Geometry check sheet. Reference: the model listing, model coordinates, mm. A direction names the side the tool comes from. Round coordinates to 2 decimals unless told otherwise and drop trailing zeros. Order: outer loops, then holes, each group sorted by start corner. A loop starts at its lowest first (then second) coordinate and runs counter-clockwise, first axis right, second up. Notation, with made-up numbers: (3, 82) -> (23, 82) arc R36 ccw to (23, 121) -> close; hole circle Ø2 at (5.25, 13). An arc over 180 degrees is marked (long way). Answer as a JSON object with one key per item and string values. Group by question number.
from build123d import *

# Parameters (mm, degrees)
EXTRUDE_1_DEPTH     = 47.7
CUT_EXTRUDE_1_DEPTH = 10
SKETCH_4_R          = 1.5
CUT_EXTRUDE_2_DEPTH = 10
SKETCH_6_R          = 2.5
CUT_EXTRUDE_4_DEPTH = 3


with BuildPart() as part:
    # 草图1 → 凸台-拉伸1 (new body)
    with BuildSketch(Plane(origin=(0, 0, 0), x_dir=(1, 0, 0), z_dir=(0, 1, 0))):
        Polygon((70.07, 0), (76.07, -6), (94.07, -6), (94.07, 0.5), (84.77, 0.5), (79.27, 6), (0, 6), (-79.27, 6), (-84.77, 0.5), (-94.07, 0.5), (-94.07, -6), (-76.07, -6), (-70.07, 0), align=None)
    extrude(amount=EXTRUDE_1_DEPTH)

    # 草图2 → 切除-拉伸1 (cut)
    with BuildSketch(Plane(origin=(0, 0, -6), x_dir=(-1, 0, 0), z_dir=(0, 0, -1))):
        Polygon((-69.27, 39.7), (-69.27, 8), (-54.27, 8), align=None)
        Polygon((-27.632185319, 39.7), (-62.632185319, 39.7), (-47.632185319, 8), align=None)
        Polygon((-40.537826527, 8), (-6.557580565, 8), (-20.537826527, 39.7), align=None)
        Polygon((-13.980245962, 39.7), (0, 8), (13.980245962, 39.7), align=None)
        Polygon((6.557580565, 8), (40.537826527, 8), (20.537826527, 39.7), align=None)
        Polygon((27.632185319, 39.7), (47.632185319, 8), (62.632185319, 39.7), align=None)
        Polygon((69.27, 39.7), (54.27, 8), (69.27, 8), align=None)
    extrude(amount=-CUT_EXTRUDE_1_DEPTH, mode=Mode.SUBTRACT)

    # 草图4 → 切除-拉伸2 (cut)
    with BuildSketch(Plane(origin=(0, 0, -0.5), x_dir=(-1, 0, 0), z_dir=(0, 0, -1))):
        with Locations((-89.57, 34.7)):
            Circle(SKETCH_4_R)
        with Locations((-89.57, 12.2)):
            Circle(SKETCH_4_R)
        with Locations((89.57, 34.7)):
            Circle(SKETCH_4_R)
        with Locations((89.57, 12.2)):
            Circle(SKETCH_4_R)
    extrude(amount=-CUT_EXTRUDE_2_DEPTH, mode=Mode.SUBTRACT)

    # 草图6 → 切除-拉伸4 (cut)
    with BuildSketch(Plane(origin=(0, 0, -0.5), x_dir=(-1, 0, 0), z_dir=(0, 0, -1))):
        with Locations((-89.57, 34.7)):
            Circle(SKETCH_6_R)
        with Locations((-89.57, 12.2)):
            Circle(SKETCH_6_R)
        with Locations((89.57, 34.7)):
            Circle(SKETCH_6_R)
        with Locations((89.57, 12.2)):
            Circle(SKETCH_6_R)
    extrude(amount=-CUT_EXTRUDE_4_DEPTH, mode=Mode.SUBTRACT)


solid = part.part
Item 1: Set-up check for faces 1 (the cylindrical face through (-87.73, 36.39, 0.98)), 2 (the flat face through (-73.11, 23.52, 3.04)), 3 (the flat face through (-30.678, 23.628, -3.042)): record each of +Z, -Z, +X, -X, +Y, -Y from which the full face is reachable in a straight line by a thin tool's end or side.
Item 2: Sectioned sample at A-A, the plane x = 24.5. Enter the section's corners in (y, z), then the cut area to 3 significant figures.
Item 3: Sectioned sample at B-B, the plane y = 29. Count the separate pieces of the cut face and the enclosed holes in it, then the cut area to 3 significant figures.
Item 4: Thickness scan on L1, parallel to Y at x = -89.57, z = 5.15; L2, parallel to Y at x = -89.57, z = 0.65; L3, parallel to X at y = 4.5, z = 4. Record the ranges inside material, lowest first.
Item 5: Depth check by flat-ended pin: pin 1 Ø6.5 at (x, y) = (89.57, 12.2) entering from -Z; pin 2 Ø5 at (x, y) = (89.57, 12.2) entering from +Z; pin 3 Ø6 at (x, y) = (-16, 26.5) entering from +Z; pin 4 Ø1.8 at (y, z) = (22, -2.5) entering from -X. Enter the tip coordinate at first touch or a pass-through.
Item 6: Mould release check, pull along Y, two halves, no side actions. Record for faces 4 (the flat face through (-91, 11, 2.5)), 5 (the flat face through (89, 24, -0.5)): pulls with the +Y half, pulls with the -Y half, needs draft (parallel to the pull), parting line crosses it, or undercut.
Result:
{
 "1": {"face 1": "-Z", "face 2": "+Z, +Y, -Y", "face 3": "+Z, -Z"},
 "2": {"outline": "(0, -6) -> (8, -6) -> (8, 0) -> (0, 0) -> close; (33.42, -6) -> (47.7, -6) -> (47.7, 0) -> (33.42, 0) -> close", "area": "134 mm2"},
 "3": {"separate pieces": "8", "enclosed holes": "0", "area": "661 mm2"},
 "4": {"L1": "y = 0 to 10.7, 13.7 to 33.2, 36.2 to 47.7", "L2": "y = 0 to 9.7, 14.7 to 32.2, 37.2 to 47.7", "L3": "x = -94.07 to -74.07, 74.07 to 94.07"},
 "5": {"pin 1": "stops at z = -0.5", "pin 2": "stops at z = 6", "pin 3": "stops at z = 0", "pin 4": "stops at x = -83.67"},
 "6": {"face 4": "undercut", "face 5": "needs draft"}
}
